Autodesk Inventor part; units mm, degrees
ref_plane "YZ Plane" through (0, 0, 0) normal (1, 0, 0) x (0, 1, 0)
ref_plane "XZ Plane" through (0, 0, 0) normal (0, 1, 0) x (-1, 0, 0)
sketch "Esboço1" plane through (0, 0, 0) normal (0, 0, 1) x (1, 0, 0)
  line L0 (0, 0) -> (107, 0)
  line L1 (0, 0) -> (2.2532, 3.75)
  line L2 (0, 0) -> (4.3749, 0) construction
  line L3 (2.2532, 3.75) -> (13, 3.75)
  line L4 (13, 3.75) -> (13, 5)
  line L5 (13, 5) -> (73, 5)
  line L6 (73, 5) -> (73, 8)
  line L7 (73, 8) -> (78, 8)
  line L8 (78, 8) -> (78, 6.5)
  line L9 (78, 6.5) -> (90, 6.5)
  line L10 (90, 6.5) -> (90, 8)
  line L11 (90, 8) -> (105, 8)
  arc A0 (107, 0) -> (105, 8) centre (90, 0) ccw
  dimension "d14" = 107
  dimension "d15" = 59
  dimension "d17" = 1.25
  dimension "d19" = 3
  dimension "d20" = 5
  dimension "d21" = 12
  dimension "d22" = 15
  dimension "d24" = 13
  dimension "d25" = 1.5
  dimension "d26" = 7.5
  dimension "d37" = 34
revolve "Revolução1" add sketch "Esboço1" angle 360 about axis through (0, 0, 0) along (1, 0, 0)
thread "Rosca1"
sketch "Esboço3" plane through (0, 0, 0) normal (0, 0, 1) x (1, 0, 0)
  circle A0 centre (98, 0) radius 3.25
  arc A1 (105, -8) -> (105, 8) centre (90, 0) ccw
  arc A2 (105, -8) -> (105, 8) centre (90, 0) ccw
  line L0 (105, -8) -> (105, 8)
  point P0 (0, 0)
  dimension "d30" = 6.5
  dimension "d34" = 7
extrude "Extrusão1" cut sketch "Esboço3" along normal through all both and the other way through all contours A0
properties part number "Parafuso2"
Here's how the part is built. I have some questions about the finished solid (model axes, mm). A direction names the side the tool comes from. Coordinates: 2 decimals unless noted, no trailing zeros. Order: outer loops, then holes, each group sorted by start corner. A loop starts at its lowest first (then second) coordinate and runs counter-clockwise, first axis right, second up. Notation, with made-up numbers: (-14.5, -28.75) - (17.5, -28.75) arc R20 ccw to (17.5, 7.25) - close; hole circle Ø3 at (83, -5). An arc over 180 degrees is marked (long way). One line per question, with ' | ' between items.
(1) If I drill on L1, parallel to Y at x = 98, z = -0.5; L2, parallel to X at y = 0, z = 0; L3, parallel to X at y = 4, z = 6.5, over which ranges is the centre line in solid material (lowest first)?
Report:
L1: y = -7.98 to -3.25, 3.25 to 7.98 | L2: x = 0 to 94.75, 101.25 to 107 | L3: x = 73 to 78, 90 to 105.19
(2) Suppose I cut it at B-B on x = 58. List the corners of the cut face in (y, z) for me.
Report:
outline: circle Ø10 at (0, 0)
(3) Suppose I cut it at A-A on x = 98. List the corners of the cut face in (y, z) for me.
Report:
outline: (-3.25, -7.31) - (-3.25, 7.31) arc R8 ccw to start; (3.25, -7.31) arc R8 ccw to (3.25, 7.31) - close
(4) If we mould it in two halves opening along X, with no side actions, what happens to faces 4 (the cylindrical face through (75.54, -1.73, -7.81)), 5 (the flat face through (78, 0, 7)), 6 (the cylindrical face through (94.753, -0.143, -0.112)), 7 (the flat face through (73, -0.1, -5.2))? For each: pulls with the +X half, pulls with the -X half, needs draft (parallel to the pull), parting line crosses it, or undercut.
Report:
face 4: needs draft | face 5: undercut | face 6: undercut | face 7: pulls with the -X half
(5) For faces 1 (the cylindrical face through (43.42, -1.08, -4.88)), 2 (the cylindrical face through (97.6, 7.39, -3.06)), 3 (the flat face through (90, 0, 7)), which set-ups out of +Z, -Z, +X, -X, +Y, -Y let a thin tool reach every point of the face, with its end or its side?
Report:
face 1: -X | face 2: +X, -X | face 3: none
(6) Will these pins go through, and if not, where does the flat tip stop? pin 1 (8 mm diameter, centred on x = 96, y = -5, fed in from -Z); pin 2 (5 mm diameter, centred on y = 2, z = -3.5, fed in from -X); pin 3 (5 mm diameter, centred on x = 88.5, z = 5, fed in from -Y).
Report:
pin 1: stops at z = -7.92 | pin 2: stops at x = 0.92 | pin 3: stops at y = -7.42
